Geometry: final body of the model. Coordinates: model frame, mm. A direction names the side the tool comes from. Give positions to 0.01 mm unless a question says otherwise; leave off trailing zeros. Write each loop counter-clockwise with the first axis right and the second up, starting at its lowest first coordinate (ties: lowest second). Pieces come first, ordered by that corner, then holes. Notation, with made-up numbers: M 45.25,-5 L 70.25,-5 A15 cw 70.25,2 Z; hole C -19.75,23 d5. An arc over 180 degrees is marked long. Use one line per item in the form item = value. Start each with the question number.
Item 1: Access query for faces 4 (the flat face through (-1, -79.012, -5)), 5 (the cylindrical face through (17.713, 59.801, -4.93)), 6 (the flat face through (47, 18, -10)), 7 (the cylindrical face through (31.35, -24.74, 0.8)), 8 (the cylindrical face through (3.159, -28.275, 0.805)). Directions: +Z, -Z, +X, -X, +Y, -Y. A direction counts if a zero-diameter tool reaches every point of the face in a straight line with its end or side. Return the directions, or none.
Item 2: Section query B-B on y = 3.5. Return loops of the section in (x, z), then the cut area to 3 significant figures.
Item 3: Pull-direction query (Y, two-part tool) for faces 1 (the flat face through (-44.49, 74.95, -5.41)), 2 (the flat face through (-44.58, -74.86, -5.41)), 3 (the cylindrical face through (-12.985, -44.458, 0.805)); classes: released by +Y, released by -Y, zero draft, split by the parting line, or undercut.
Item 4: Section query A-A on z = -6.75. Give the number of separate pieces and of enclosed holes in the cut face, then the cut area to 3 significant figures.
Item 5: Material intervals for line 1 along X through (y, z) = (-7.5, -3.5); line 2 along Y through (x, z) = (5, -4); line 3 along Y through (x, z) = (11, -1), sorted ascending. Write a range as from..to.
Item 6: Contact query for flat-ended pins moving along their axis: P1, Ø0.8, axis at y = -52.5, z = 0.5, coming from the -X side (3 decimals); P2, Ø5, axis at x = 10.54, y = -21.07, coming from the -Z side; P3, Ø1.7, axis at y = -30.5, z = 1, coming from the -X side (3 decimals); P4, Ø1.3, axis at x = -21, z = 1, coming from the +Y side. Output: stop coordinate, or through.
Item 7: Section query C-C on x = 2.5. Return loops of the section in (y, z).
from build123d import *

# Parameters (mm, degrees)
F3_DEPTH  = 1.5875
F1_R      = 5.08
F1_R_2    = 1.5875
F4_DEPTH  = 10
F5_DEPTH  = 10
F6_R      = 3.96875
F7_DEPTH  = 1.5875
F8_R      = 3.175
F9_DEPTH  = 11.5885
F10_SIZE  = 2.54
F11_F1_R  = 2.54
F11_F2_R  = 2.54
F11_F3_R  = 2.54
F11_F4_R  = 2.54
F11_F5_R  = 2.54
F11_F6_R  = 2.54
F11_F7_R  = 2.54
F11_F8_R  = 2.54
F11_F9_R  = 2.54
F11_F10_R = 2.54
F11_F11_R = 2.54
F11_F12_R = 2.54
F11_F13_R = 2.54
F11_F14_R = 2.54
F11_F15_R = 2.54
F11_F16_R = 2.54


with BuildPart() as f3:
    # F0 (on Top) → F3 (new body)
    with BuildSketch(Plane.XY):
        Polygon((-40.4276280605, 79.0125), (-48.6375, 70.8026280605), (-48.6375, -70.8026280605), (-40.4276280605, -79.0125), (40.4276280605, -79.0125), (48.6375, -70.8026280605), (48.6375, 70.8026280605), (40.4276280605, 79.0125), align=None)
        Polygon((-45.4625, 69.4875), (-39.1125, 75.8375), (39.1125, 75.8375), (45.4625, 69.4875), (45.4625, -69.4875), (39.1125, -75.8375), (-39.1125, -75.8375), (-45.4625, -69.4875), align=None, mode=Mode.SUBTRACT)
        Polygon((39.1125, 75.8375), (-39.1125, 75.8375), (-45.4625, 69.4875), (-45.4625, -69.4875), (-39.1125, -75.8375), (39.1125, -75.8375), (45.4625, -69.4875), (45.4625, 69.4875), align=None)
    extrude(amount=F3_DEPTH)

    # F1 (on Top) → F4 (join)
    with BuildSketch(Plane.XY):
        with Locations((27.6825, -23.2224922)):
            Circle(F1_R)
        with Locations((27.6825, -23.2224922)):
            Circle(F1_R_2, mode=Mode.SUBTRACT)
        with Locations((14.9825, 55.5175)):
            Circle(F1_R)
        with Locations((14.9825, 55.5175)):
            Circle(F1_R_2, mode=Mode.SUBTRACT)
        with Locations((-20.0625, 55.5175)):
            Circle(F1_R)
        with Locations((-20.0625, 55.5175)):
            Circle(F1_R_2, mode=Mode.SUBTRACT)
    extrude(amount=-F4_DEPTH)

    # F0 (on Top) → F5 (join)
    with BuildSketch(Plane.XY):
        Polygon((-40.4276280605, 79.0125), (-48.6375, 70.8026280605), (-48.6375, -70.8026280605), (-40.4276280605, -79.0125), (40.4276280605, -79.0125), (48.6375, -70.8026280605), (48.6375, 70.8026280605), (40.4276280605, 79.0125), align=None)
        Polygon((-45.4625, 69.4875), (-39.1125, 75.8375), (39.1125, 75.8375), (45.4625, 69.4875), (45.4625, -69.4875), (39.1125, -75.8375), (-39.1125, -75.8375), (-45.4625, -69.4875), align=None, mode=Mode.SUBTRACT)
    extrude(amount=-F5_DEPTH)

    # F6 (on face) → F7 (cut)
    with BuildSketch(Plane.XY.offset(1.5875)):
        with Locations((-20.0625, 55.5175)):
            Circle(F6_R)
        with Locations((14.9825, 55.5175)):
            Circle(F6_R)
        with Locations((27.6825, -23.2224922)):
            Circle(F6_R)
    extrude(amount=-F7_DEPTH, mode=Mode.SUBTRACT)

    # F8 (on face) → F9 (cut, through all)
    with BuildSketch(Plane.XY.offset(1.5875)):
        with Locations((-22.00625, -21.06875)):
            Circle(F8_R)
        with Locations((10.5375, -21.06875)):
            Circle(F8_R)
        with Locations((10.5375, -53.6125)):
            Circle(F8_R)
        with Locations((-22.00625, -53.6125)):
            Circle(F8_R)
        with BuildLine():
            Line((-18.3707154513, -38.610625), (-22.5138820324, -38.610625))
            ThreePointArc((-22.5138820324, -38.610625), (-17.6332143604, -49.2394643604), (-7.004375, -54.1201320324))
            Line((-7.004375, -54.1201320324), (-7.004375, -49.9769654513))
            ThreePointArc((-7.004375, -49.9769654513), (-14.7146311211, -46.3208811211), (-18.3707154513, -38.610625))
        make_face()
        with BuildLine():
            ThreePointArc((-8.6443105663, -36.070625), (-7.9794390303, -35.0955609697), (-7.004375, -34.4306894337))
            Line((-7.004375, -34.4306894337), (-7.004375, -27.2603125048))
            ThreePointArc((-7.004375, -27.2603125048), (-12.9185798969, -30.1564201031), (-15.8146874952, -36.070625))
            Line((-15.8146874952, -36.070625), (-8.6443105663, -36.070625))
        make_face()
        with BuildLine():
            Line((-4.464375, -27.2603125048), (-4.464375, -34.4306894337))
            ThreePointArc((-4.464375, -34.4306894337), (-3.4893109697, -35.0955609697), (-2.8244394337, -36.070625))
            Line((-2.8244394337, -36.070625), (4.3459374952, -36.070625))
            ThreePointArc((4.3459374952, -36.070625), (1.4498298969, -30.1564201031), (-4.464375, -27.2603125048))
        make_face()
        with BuildLine():
            Line((4.3459374952, -38.610625), (-2.8244394337, -38.610625))
            ThreePointArc((-2.8244394337, -38.610625), (-3.4893109697, -39.5856890303), (-4.464375, -40.2505605663))
            Line((-4.464375, -40.2505605663), (-4.464375, -47.4209374952))
            ThreePointArc((-4.464375, -47.4209374952), (1.4498298969, -44.5248298969), (4.3459374952, -38.610625))
        make_face()
        with BuildLine():
            Line((-7.004375, -47.4209374952), (-7.004375, -40.2505605663))
            ThreePointArc((-7.004375, -40.2505605663), (-7.9794390303, -39.5856890303), (-8.6443105663, -38.610625))
            Line((-8.6443105663, -38.610625), (-15.8146874952, -38.610625))
            ThreePointArc((-15.8146874952, -38.610625), (-12.9185798969, -44.5248298969), (-7.004375, -47.4209374952))
        make_face()
        with BuildLine():
            Line((-22.5138820324, -36.070625), (-18.3707154513, -36.070625))
            ThreePointArc((-18.3707154513, -36.070625), (-14.7146311211, -28.3603688789), (-7.004375, -24.7042845487))
            Line((-7.004375, -24.7042845487), (-7.004375, -20.5611179676))
            ThreePointArc((-7.004375, -20.5611179676), (-17.6332143604, -25.4417856396), (-22.5138820324, -36.070625))
        make_face()
        with BuildLine():
            ThreePointArc((-4.464375, -24.7042845487), (3.2458811211, -28.3603688789), (6.9019654513, -36.070625))
            Line((6.9019654513, -36.070625), (11.0451320324, -36.070625))
            ThreePointArc((11.0451320324, -36.070625), (6.1644643604, -25.4417856396), (-4.464375, -20.5611179676))
            Line((-4.464375, -20.5611179676), (-4.464375, -24.7042845487))
        make_face()
        with BuildLine():
            Line((11.0451320324, -38.610625), (6.9019654513, -38.610625))
            ThreePointArc((6.9019654513, -38.610625), (3.2458811211, -46.3208811211), (-4.464375, -49.9769654513))
            Line((-4.464375, -49.9769654513), (-4.464375, -54.1201320324))
            ThreePointArc((-4.464375, -54.1201320324), (6.1644643604, -49.2394643604), (11.0451320324, -38.610625))
        make_face()
    extrude(amount=-F9_DEPTH, mode=Mode.SUBTRACT)

    # F10
    f10_edges = [f3.edges().sort_by_distance(p)[0] for p in [
        (0, 79.0125, 1.5875),
        (-44.532564, 74.907564, 1.5875),
        (-48.6375, 0, 1.5875),
        (44.532564, 74.907564, 1.5875),
        (48.6375, 0, 1.5875),
        (-44.532564, -74.907564, 1.5875),
        (0, -79.0125, 1.5875),
        (44.532564, -74.907564, 1.5875),
    ]]
    chamfer(f10_edges, length=F10_SIZE)

    # F11: fillet of radius 2.54 on 16 edges, made by hand

    # F11_f1
    f11_f1_edges = [f3.edges().sort_by_distance(p)[0] for p in [
        (-40.4276280605, 79.0125, -5.47625),
    ]]
    fillet(f11_f1_edges, radius=F11_F1_R)

    # F11_f2
    f11_f2_edges = [f3.edges().sort_by_distance(p)[0] for p in [
        (-48.6375, 70.8026280605, -5.47625),
    ]]
    fillet(f11_f2_edges, radius=F11_F2_R)

    # F11_f3
    f11_f3_edges = [f3.edges().sort_by_distance(p)[0] for p in [
        (40.4276280605, 79.0125, -5.47625),
    ]]
    fillet(f11_f3_edges, radius=F11_F3_R)

    # F11_f4
    f11_f4_edges = [f3.edges().sort_by_distance(p)[0] for p in [
        (-39.8615335712, 77.6458270063, 0.4141729937),
    ]]
    fillet(f11_f4_edges, radius=F11_F4_R)

    # F11_f5
    f11_f5_edges = [f3.edges().sort_by_distance(p)[0] for p in [
        (-47.2708270063, 70.2365335712, 0.4141729937),
    ]]
    fillet(f11_f5_edges, radius=F11_F5_R)

    # F11_f6
    f11_f6_edges = [f3.edges().sort_by_distance(p)[0] for p in [
        (-48.6375, -70.8026280605, -5.47625),
    ]]
    fillet(f11_f6_edges, radius=F11_F6_R)

    # F11_f7
    f11_f7_edges = [f3.edges().sort_by_distance(p)[0] for p in [
        (48.6375, 70.8026280605, -5.47625),
    ]]
    fillet(f11_f7_edges, radius=F11_F7_R)

    # F11_f8
    f11_f8_edges = [f3.edges().sort_by_distance(p)[0] for p in [
        (39.8615335712, 77.6458270063, 0.4141729937),
    ]]
    fillet(f11_f8_edges, radius=F11_F8_R)

    # F11_f9
    f11_f9_edges = [f3.edges().sort_by_distance(p)[0] for p in [
        (-47.2708270063, -70.2365335712, 0.4141729937),
    ]]
    fillet(f11_f9_edges, radius=F11_F9_R)

    # F11_f10
    f11_f10_edges = [f3.edges().sort_by_distance(p)[0] for p in [
        (-40.4276280605, -79.0125, -5.47625),
    ]]
    fillet(f11_f10_edges, radius=F11_F10_R)

    # F11_f11
    f11_f11_edges = [f3.edges().sort_by_distance(p)[0] for p in [
        (40.4276280605, -79.0125, -5.47625),
    ]]
    fillet(f11_f11_edges, radius=F11_F11_R)

    # F11_f12
    f11_f12_edges = [f3.edges().sort_by_distance(p)[0] for p in [
        (48.6375, -70.8026280605, -5.47625),
    ]]
    fillet(f11_f12_edges, radius=F11_F12_R)

    # F11_f13
    f11_f13_edges = [f3.edges().sort_by_distance(p)[0] for p in [
        (47.2708270063, 70.2365335712, 0.4141729937),
    ]]
    fillet(f11_f13_edges, radius=F11_F13_R)

    # F11_f14
    f11_f14_edges = [f3.edges().sort_by_distance(p)[0] for p in [
        (47.2708270063, -70.2365335712, 0.4141729937),
    ]]
    fillet(f11_f14_edges, radius=F11_F14_R)

    # F11_f15
    f11_f15_edges = [f3.edges().sort_by_distance(p)[0] for p in [
        (39.8615335712, -77.6458270063, 0.4141729937),
    ]]
    fillet(f11_f15_edges, radius=F11_F15_R)

    # F11_f16
    f11_f16_edges = [f3.edges().sort_by_distance(p)[0] for p in [
        (-39.8615335712, -77.6458270063, 0.4141729937),
    ]]
    fillet(f11_f16_edges, radius=F11_F16_R)


solid = f3.part
Answer sheet:
q1.face_4 = +Z, -Z, +X, -X, -Y
q1.face_5 = -Z
q1.face_6 = -Z, +X, -X, +Y, -Y
q1.face_7 = +Z
q1.face_8 = +Z, -Z
q2.outline = M -48.64,-10 L -45.46,-10 L -45.46,0 L 45.46,0 L 45.46,-10 L 48.64,-10 L 48.64,-0.95 L 46.1,1.59 L -46.1,1.59 L -48.64,-0.95 Z
q2.area = 211 mm2
q3.face_1 = released by +Y
q3.face_2 = released by -Y
q3.face_3 = undercut
q4.separate_pieces = 4
q4.enclosed_holes = 4
q4.area = 1,750 mm2
q5.line_1 = -48.64..-45.46, 45.46..48.64
q5.line_2 = -79.01..-75.84, 75.84..79.01
q5.line_3 = -79.01..-75.84, 52.36..58.67, 75.84..79.01
q6.P1 = -47.585
q6.P2 = through
q6.P3 = -47.535
q6.P4 = 77.71
q7.outline = M -79.01,-10 L -75.84,-10 L -75.84,0 L -52.02,0 L -52.02,1.59 L -76.47,1.59 L -79.01,-0.95 Z; M -47.01,0 L -43.29,0 L -43.29,1.59 L -47.01,1.59 Z; M -38.61,0 L -36.07,0 L -36.07,1.59 L -38.61,1.59 Z; M -31.39,0 L -27.67,0 L -27.67,1.59 L -31.39,1.59 Z; M -22.67,0 L 75.84,0 L 75.84,-10 L 79.01,-10 L 79.01,-0.95 L 76.47,1.59 L -22.67,1.59 Z
